from build123d import *

# Parameters (mm, degrees)
F0_W     = 228.000006
F0_H     = 128.000006
F1_DEPTH = 3


with BuildPart() as f1:
    # F0 (on Front) → F1 (new body)
    with BuildSketch(Plane.XZ):
        Rectangle(F0_W, F0_H)
        with BuildLine():
            Line((100, -35.578923), (100, -50))
            Line((100, -50), (70.984792, -50))
            Line((70.984792, -50), (29.015208, -50))
            Line((29.015208, -50), (-29.015208, -50))
            Line((-29.015208, -50), (-70.984792, -50))
            Line((-70.984792, -50), (-100, -50))
            Line((-100, -50), (-100, -35.578923))
            Line((-100, -35.578923), (-100, 34.356112))
            Line((-100, 34.356112), (-100, 50))
            Line((-100, 50), (-70.984792, 50))
            Line((-70.984792, 50), (-29.015208, 50))
            Line((-29.015208, 50), (18.414966, 50))
            Line((18.414966, 50), (29.015208, 50))
            Line((29.015208, 50), (70.984792, 50))
            Line((70.984792, 50), (81.585034, 50))
            Line((81.585034, 50), (100, 50))
            Line((100, 50), (100, 37.225828))
            Line((100, 37.225828), (100.116007, -34.500008))
            ThreePointArc((100.116007, -34.500008), (100.087359, -35.042622), (100, -35.578923))
        make_face(mode=Mode.SUBTRACT)
        with BuildLine():
            Line((70.984792, -50), (100, -50))
            Line((100, -50), (100, -35.578923))
            ThreePointArc((100, -35.578923), (96.197739, -39.38968), (91.141582, -37.541887))
            Line((91.141582, -37.541887), (64.800607, -3.033792))
            ThreePointArc((64.800607, -3.033792), (63.775038, 0), (64.800607, 3.033792))
            Line((64.800607, 3.033792), (91.025569, 37.389904))
            ThreePointArc((91.025569, 37.389904), (96.601225, 39.092785), (100, 34.356112))
            Line((100, 34.356112), (100, 37.225828))
            Line((100, 37.225828), (100, 50))
            Line((100, 50), (81.585034, 50))
            Line((81.585034, 50), (70.984792, 50))
            ThreePointArc((70.984792, 50), (75.466363, 47.217097), (74.959223, 41.966208))
            Line((74.959223, 41.966208), (53.974431, 14.475001))
            ThreePointArc((53.974431, 14.475001), (50, 12.508793), (46.025569, 14.475001))
            Line((46.025569, 14.475001), (25.040777, 41.966208))
            ThreePointArc((25.040777, 41.966208), (24.533637, 47.217097), (29.015208, 50))
            Line((29.015208, 50), (18.414966, 50))
            Line((18.414966, 50), (-29.015208, 50))
            ThreePointArc((-29.015208, 50), (-24.533637, 47.217097), (-25.040777, 41.966208))
            Line((-25.040777, 41.966208), (-46.025569, 14.475001))
            ThreePointArc((-46.025569, 14.475001), (-50, 12.508793), (-53.974431, 14.475001))
            Line((-53.974431, 14.475001), (-74.959223, 41.966208))
            ThreePointArc((-74.959223, 41.966208), (-75.466363, 47.217097), (-70.984792, 50))
            Line((-70.984792, 50), (-100, 50))
            Line((-100, 50), (-100, 34.356112))
            ThreePointArc((-100, 34.356112), (-96.601225, 39.092785), (-91.025569, 37.389904))
            Line((-91.025569, 37.389904), (-64.800607, 3.033792))
            ThreePointArc((-64.800607, 3.033792), (-63.775038, 0), (-64.800607, -3.033792))
            Line((-64.800607, -3.033792), (-91.141582, -37.541887))
            ThreePointArc((-91.141582, -37.541887), (-96.197739, -39.38968), (-100, -35.578923))
            Line((-100, -35.578923), (-100, -50))
            Line((-100, -50), (-70.984792, -50))
            ThreePointArc((-70.984792, -50), (-75.466363, -47.217097), (-74.959223, -41.966208))
            Line((-74.959223, -41.966208), (-53.974431, -14.475001))
            ThreePointArc((-53.974431, -14.475001), (-50, -12.508793), (-46.025569, -14.475001))
            Line((-46.025569, -14.475001), (-25.040777, -41.966208))
            ThreePointArc((-25.040777, -41.966208), (-24.533637, -47.217097), (-29.015208, -50))
            Line((-29.015208, -50), (29.015208, -50))
            ThreePointArc((29.015208, -50), (24.533637, -47.217097), (25.040777, -41.966208))
            Line((25.040777, -41.966208), (46.025569, -14.475001))
            ThreePointArc((46.025569, -14.475001), (50, -12.508793), (53.974431, -14.475001))
            Line((53.974431, -14.475001), (74.959223, -41.966208))
            ThreePointArc((74.959223, -41.966208), (75.466363, -47.217097), (70.984792, -50))
        make_face()
        with BuildLine():
            Line((24.959223, -17.302074), (3.974431, -44.793281))
            ThreePointArc((3.974431, -44.793281), (0, -46.759489), (-3.974431, -44.793281))
            Line((-3.974431, -44.793281), (-24.959223, -17.302074))
            ThreePointArc((-24.959223, -17.302074), (-25.466363, -12.051185), (-20.984792, -9.268282))
            Line((-20.984792, -9.268282), (0, -9.268282))
            Line((0, -9.268282), (20.984792, -9.268282))
            ThreePointArc((20.984792, -9.268282), (25.466363, -12.051185), (24.959223, -17.302074))
        make_face(mode=Mode.SUBTRACT)
        with BuildLine():
            ThreePointArc((-3.974431, 44.793281), (0, 46.759489), (3.974431, 44.793281))
            Line((3.974431, 44.793281), (24.959223, 17.302074))
            ThreePointArc((24.959223, 17.302074), (25.466363, 12.051185), (20.984792, 9.268282))
            Line((20.984792, 9.268282), (0, 9.268282))
            Line((0, 9.268282), (-20.984792, 9.268282))
            ThreePointArc((-20.984792, 9.268282), (-25.466363, 12.051185), (-24.959223, 17.302074))
            Line((-24.959223, 17.302074), (-3.974431, 44.793281))
        make_face(mode=Mode.SUBTRACT)
    extrude(amount=F1_DEPTH)


solid = f1.part
CAD build for the part. Positions are in the model's coordinates, mm. Coordinates: 2 decimals unless noted, no trailing zeros. Write each loop counter-clockwise with the first axis right and the second up, starting at its lowest first coordinate (ties: lowest second). Pieces come first, ordered by that corner, then holes. Notation, with made-up numbers: M 73.5,52 L 87.5,52 A11 ccw 87.5,70 Z; hole C 27,30.25 d9. An arc over 180 degrees is marked long. Return JSON: item names as keys, results as strings.
Item 1: Slice it at D-D, the plane y = -0.8. State how many separate pieces and enclosed holes the cut face has, and give its area (3 significant figures).
Findings below:
{"separate pieces": "1", "enclosed holes": "8", "area": "18,400 mm2"}
Item 2: Slice it at A-A, the plane x = 1. Write the cut outline in (y, z).
Findings below:
{"outline": "M -3,-64 L 0,-64 L 0,-46.66 L -3,-46.66 Z; M -3,-9.27 L 0,-9.27 L 0,9.27 L -3,9.27 Z; M -3,46.66 L 0,46.66 L 0,64 L -3,64 Z"}
Item 3: Slice it at C-C, the plane z = -32. Write the cut outline in (x, y).
Findings below:
{"outline": "M -114,-3 L -100,-3 L -100,0 L -114,0 Z; M -86.91,-3 L -67.35,-3 L -67.35,0 L -86.91,0 Z; M -32.65,-3 L -13.74,-3 L -13.74,0 L -32.65,0 Z; M 13.74,-3 L 32.65,-3 L 32.65,0 L 13.74,0 Z; M 67.35,-3 L 86.91,-3 L 86.91,0 L 67.35,0 Z; M 100.11,-3 L 114,-3 L 114,0 L 100.11,0 Z"}
Item 4: Drop a flat-ended pin along its axis: pin 1 Ø1.5 at (x, z) = (24.5, 45) entering from +Y. Give the stop position or say it passes through.
Findings below:
{"pin 1": "stops at y = 0"}
Item 5: Two-plate mould, pull along Z, no slides. Class faces 1 (the cylindrical face through (-96.684, -1.479, 39.064)), 2 (the cylindrical face through (24.5, -1.48, 47.15)), 3 (the flat face through (-27, 0, 1)): +Z half, -Z half, draft (parallel to the pull), parting line (faces both ways), or undercut.
Findings below:
{"face 1": "undercut", "face 2": "undercut", "face 3": "draft"}
Item 6: Probe line 1 (X direction, y = -2.55, z = 49); line 2 (Z direction, x = 63, y = -1.4); line 3 (Z direction, x = -46, y = -1.95). List the from-to ranges inside material, lowest first. Write a range as from..to.
Findings below:
{"line 1": "x = -114..-73.98, -26.02..26.02, 73.98..114", "line 2": "z = -64..-50, -26.3..26.3, 50..64", "line 3": "z = -64..-50, -14.51..14.51, 50..64"}
Item 7: Slice it at B-B, the plane z = 7. Write the cut outline in (x, y), and give its area (3 significant figures).
Findings below:
{"outline": "M -114,-3 L -100,-3 L -100,0 L -114,0 Z; M -67.83,-3 L 67.83,-3 L 67.83,0 L -67.83,0 Z; M 100.05,-3 L 114,-3 L 114,0 L 100.05,0 Z", "area": "491 mm2"}
